Here's how the part is built. I have some questions about the finished solid (model axes, mm). A direction names the side the tool comes from. Coordinates: 2 decimals unless noted, no trailing zeros. Write each loop counter-clockwise with the first axis right and the second up, starting at its lowest first coordinate (ties: lowest second). Pieces come first, ordered by that corner, then holes.
Item 1: If we section it at C-C (y = 0.45): Please give me the cut outline in (x, z).
Item 2: For faces 1 (the face through (0, 1, -21)), 2 (the face through (-1, 0, 9)), which set-ups out of +Z, -Z, +X, -X, +Y, -Y let a thin tool reach every point of the face, with its end or its side?
Item 3: If we section it at A-A (x = 0): Please give me the cut outline in (y, z), then the cut area to 3 significant figures.
Item 4: I'm going to push a flat-ended pin straight in: pin 1 Ø6 at (x, z) = (-15, -8.5) entering from -Y. Where does the tip first touch, or does it pass through?
Item 5: If we section it at B-B (z = 0): Please give me the cut outline in (x, y), then the cut area to 3 significant figures.
Item 6: If we section it at D-D (z = 12.5): Please give me the cut outline in (x, y).
Item 7: If I drill on line 1 (X direction, y = 1.4, z = 0); line 2 (X direction, y = 0.4, z = -12); line 3 (X direction, y = 0.4, z = 12), over which ranges is the centre line in solid material (lowest first)?
Item 8: We'd pull the mould along X, two halves only. Please class faces 3 (the face through (11.685, 0.986, -8.806)), 4 (the face through (0, 1, 6)), 5 (the face through (-40, 1, -9)), 6 (the face through (-1, 2, 9)): +X half, -X half, draft (parallel to the pull), parting line (faces both ways), or undercut.
from build123d import *

# Parameters (mm, degrees)
SKETCH1_R           = 41
BOSS_EXTRUDE1_DEPTH = 2


with BuildPart() as part:
    # Sketch1 → Boss-Extrude1 (new body)
    # profile 1 of 2: a face of its own
    with BuildSketch(Plane(origin=(0, 0, 0), x_dir=(1, 0, 0), z_dir=(0, 1, 0))):
        with Locations(Location((0, 0, 0), (0, 0, 270))):
            Circle(SKETCH1_R)
        with BuildLine():
            ThreePointArc((21, 0), (-9.127670618, -18.912578594), (-13.065298009, 16.440741709))
            ThreePointArc((-13.065298009, 16.440741709), (-12.557369181, 16.831888761), (-12.037737576, 17.20734942))
            ThreePointArc((-12.037737576, 17.20734942), (0, 21), (12.037737576, 17.20734942))
            ThreePointArc((12.037737576, 17.20734942), (12.557369181, 16.831888761), (13.065298009, 16.440741709))
            ThreePointArc((13.065298009, 16.440741709), (18.912578594, 9.127670618), (21, 0))
        make_face(mode=Mode.SUBTRACT)
    # profile 2 of 2: a face of its own
    with BuildSketch(Plane(origin=(0, 0, 0), x_dir=(1, 0, 0), z_dir=(0, 1, 0))):
        with BuildLine():
            ThreePointArc((-12.037737576, 17.20734942), (-12.557369181, 16.831888761), (-13.065298009, 16.440741709))
            ThreePointArc((-13.065298009, 16.440741709), (-9.127670618, -18.912578594), (21, 0))
            ThreePointArc((21, 0), (18.912578594, 9.127670618), (13.065298009, 16.440741709))
            ThreePointArc((13.065298009, 16.440741709), (12.557369181, 16.831888761), (12.037737576, 17.20734942))
            ThreePointArc((12.037737576, 17.20734942), (11.628117295, 8.696683132), (4.806650128, 3.591116059))
            ThreePointArc((4.806650128, 3.591116059), (0, -6), (-4.806650128, 3.591116059))
            ThreePointArc((-4.806650128, 3.591116059), (-11.628117295, 8.696683132), (-12.037737576, 17.20734942))
        make_face()
    extrude(amount=BOSS_EXTRUDE1_DEPTH)


solid = part.part
Answer list:
1. outline: circle Ø82 at (0, 0); hole (-12.04, -17.21) arc R21 ccw to (12.04, -17.21) arc R10 ccw to (4.81, -3.59) arc R6 ccw (long way) to (-4.81, -3.59) arc R10 ccw to start
2. face 1: +Y, -Y
2. face 2: +Z, -Z, +X, -X, -Y
3. outline: (0, -41) - (2, -41) - (2, -21) - (0, -21) - close; (0, 6) - (2, 6) - (2, 41) - (0, 41) - close
3. area: 110 mm2
4. pin 1: stops at y = 0
5. outline: (-41, 0) - (-6, 0) - (-6, 2) - (-41, 2) - close; (6, 0) - (41, 0) - (41, 2) - (6, 2) - close
5. area: 140 mm2
6. outline: (-39.05, 0) - (39.05, 0) - (39.05, 2) - (-39.05, 2) - close
7. line 1: x = -41 to -6, 6 to 41
7. line 2: x = -39.2 to -12.7, 12.7 to 39.2
7. line 3: x = -39.2 to 39.2
8. face 3: undercut
8. face 4: undercut
8. face 5: parting line
8. face 6: draft
